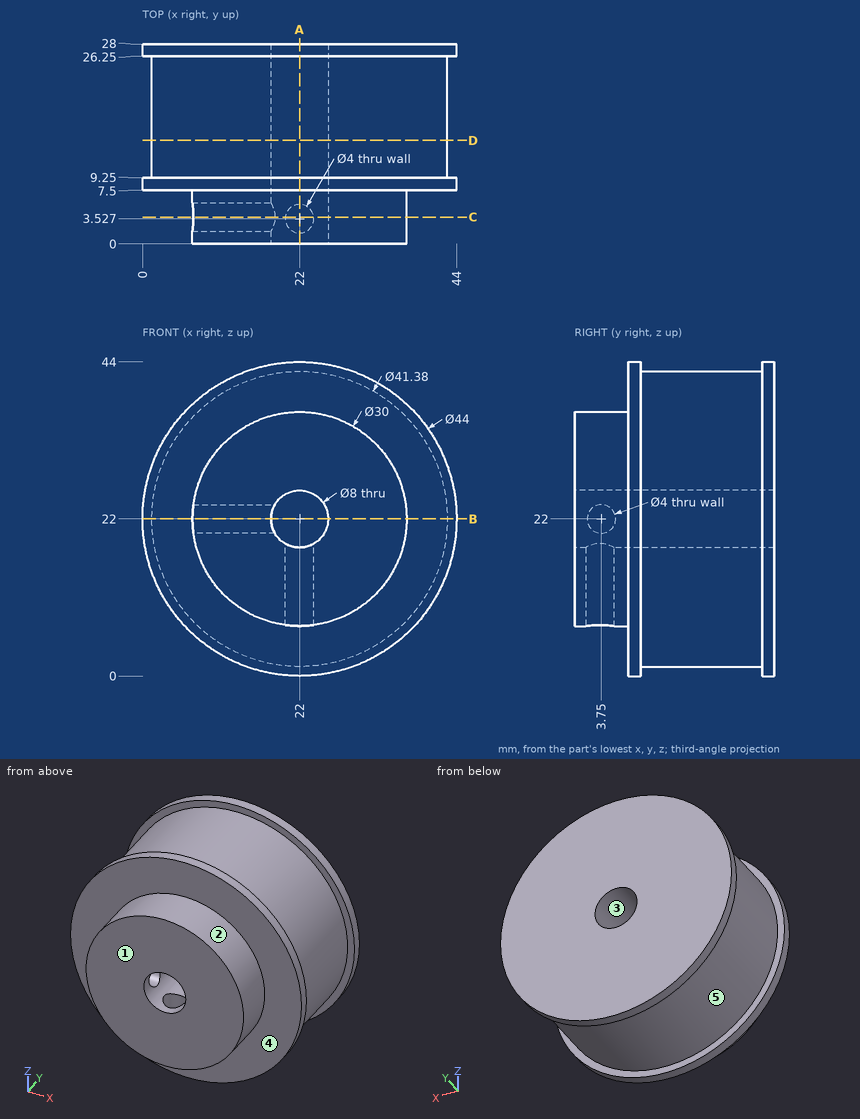
Check sheet for the drawn part. Datum: minimum x, y, z corner. Units: mm. A direction names the side the tool comes from. Coordinates: 2 decimals unless noted, no trailing zeros. Write each loop counter-clockwise with the first axis right and the second up, starting at its lowest first coordinate (ties: lowest second). Pieces come first, ordered by that corner, then holes. Notation, with made-up numbers: (8.5, -15.5) - (29.5, -15.5) arc R26 cw to (29.5, 21.5) - close; hole circle Ø8 at (-9, 37). An arc over 180 degrees is marked (long way). Answer as a JSON object with one key per item and string values.
(1) Thickness scan on line 1 along X through (y, z) = (6.75, 22); line 2 along X through (y, z) = (15, 22); line 3 along Y through (x, z) = (10.5, 11). Record the ranges inside material, lowest first.
Report:
{"line 1": "7 to 18, 26 to 37", "line 2": "1.31 to 18, 26 to 42.69", "line 3": "7.5 to 28"}
(2) Gauge pin test, flat ends, axial feed: pin 1 Ø2.5 at (y, z) = (3.75, 22) entering from +X; pin 2 Ø1 at (x, y) = (8.5, 6) entering from +Z (1 decimal); pin 3 Ø7 at (x, z) = (22, 22) entering from -Y; pin 4 Ø6 at (x, y) = (32, 23) entering from -Z. Record the tip position at first contact, or that the pin passes through.
Report:
{"pin 1": "x = 37", "pin 2": "z = 29.5", "pin 3": "through", "pin 4": "z = 2.53"}
(3) Tool access check on the marked faces 1 and 2. Record the directions out of +Z, -Z, +X, -X, +Y, -Y that give a thin tool (end or side, any length) a straight path to the whole face; none if there is none.
Report:
{"face 1": "+Z, -Z, +X, -X, -Y", "face 2": "-Y"}
(4) Cross-section at A-A on x = 22. Record the cut outline in (y, z).
Report:
{"outline": "(0, 7) - (1.53, 7) - (1.53, 18) - (0, 18) - close; (0, 26) - (28, 26) - (28, 44) - (26.25, 44) - (26.25, 42.69) - (9.25, 42.69) - (9.25, 44) - (7.5, 44) - (7.5, 37) - (0, 37) - close; (5.53, 7) - (7.5, 7) - (7.5, 0) - (9.25, 0) - (9.25, 1.31) - (26.25, 1.31) - (26.25, 0) - (28, 0) - (28, 18) - (5.53, 18) - close"}
(5) Cross-section at B-B on z = 22. Record the cut outline in (x, y).
Report:
{"outline": "(0, 7.5) - (7, 7.5) - (7, 5.75) - (18, 5.75) - (18, 28) - (0, 28) - (0, 26.25) - (1.31, 26.25) - (1.31, 9.25) - (0, 9.25) - close; (7, 0) - (18, 0) - (18, 1.75) - (7, 1.75) - close; (26, 0) - (37, 0) - (37, 7.5) - (44, 7.5) - (44, 9.25) - (42.69, 9.25) - (42.69, 26.25) - (44, 26.25) - (44, 28) - (26, 28) - close"}
(6) Cross-section at D-D on y = 14.5. Record the cut outline in (x, z).
Report:
{"outline": "circle Ø41.38 at (22, 22); hole circle Ø8 at (22, 22)"}
(7) Cross-section at C-C on y = 3.75. Record the cut outline in (x, z).
Report:
{"outline": "(7.13, 20) arc R15 ccw to (20.01, 7.13) - (20.01, 18.53) arc R4 cw to (18.54, 20) - close; (7.13, 24) - (18.54, 24) arc R4 cw (long way) to (23.99, 18.53) - (23.99, 7.13) arc R15 ccw (long way) to start"}
(8) Mould release check, pull along X, two halves, no side actions. Record for the marked faces 3, 4 and 5: pulls with the +X half, pulls with the -X half, needs draft (parallel to the pull), parting line crosses it, or undercut.
Report:
{"face 3": "undercut", "face 4": "needs draft", "face 5": "parting line crosses it"}
